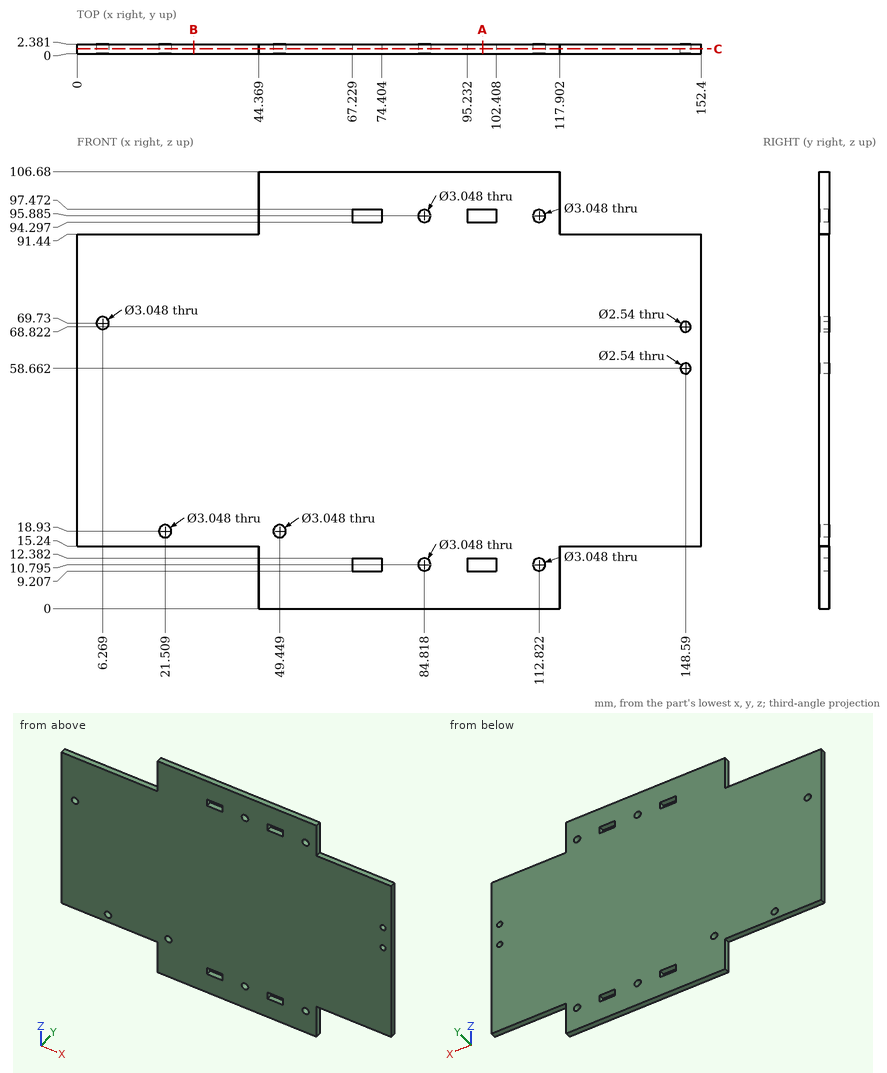
Check sheet for the drawn part. Datum: minimum x, y, z corner. Units: mm. Round coordinates to 2 decimals unless told otherwise and drop trailing zeros. Loops run counter-clockwise (first coordinate to the right, second up) from the corner with the lowest first, then second, coordinate; pieces in that order, holes last. Notation, with made-up numbers: M 16.25,-39 L 58.25,-39 A11 ccw 58.25,-24 Z; hole C -25.75,5.25 d9. An arc over 180 degrees is marked long. Write each question's results on one line, items separated by ' | '.
1) Scan lines: L1, parallel to Z at x = 96, y = 0.1; L2, parallel to Z at x = 85, y = 0.8; L3, parallel to X at y = 0.8, z = 92.5. Record each from-to range of solid material in increasing order. Write a range as from..to.
Checks:
L1: z = 0..9.21, 12.38..94.3, 97.47..106.68 | L2: z = 0..9.28, 12.31..94.37, 97.4..106.68 | L3: x = 44.37..117.9
2) Gauge pin test, flat ends, axial feed: P1, Ø0.7, axis at y = 0.5, z = 11.5, coming from the +X side; P2, Ø0.7, axis at y = 1.5, z = 10.5, coming from the -X side. Record the tip position at first contact, or that the pin passes through.
Checks:
P1: stops at x = 117.9 | P2: stops at x = 44.37
3) Section check C-C on y = 1.2. State how many separate pieces and enclosed holes the cut face has, then the cut area to 3 significant figures.
Checks:
separate pieces: 1 | enclosed holes: 13 | area: 13,700 mm2
4) Section check A-A on x = 99. Record the boundary of the cut face in (y, z), then the cut area to 3 significant figures.
Checks:
outline: M 0,0 L 2.38,0 L 2.38,9.21 L 0,9.21 Z; M 0,12.38 L 2.38,12.38 L 2.38,94.3 L 0,94.3 Z; M 0,97.47 L 2.38,97.47 L 2.38,106.68 L 0,106.68 Z | area: 239 mm2
5) Section check B-B on x = 28.5. Record the boundary of the cut face in (y, z).
Checks:
outline: M 0,15.24 L 2.38,15.24 L 2.38,91.44 L 0,91.44 Z
